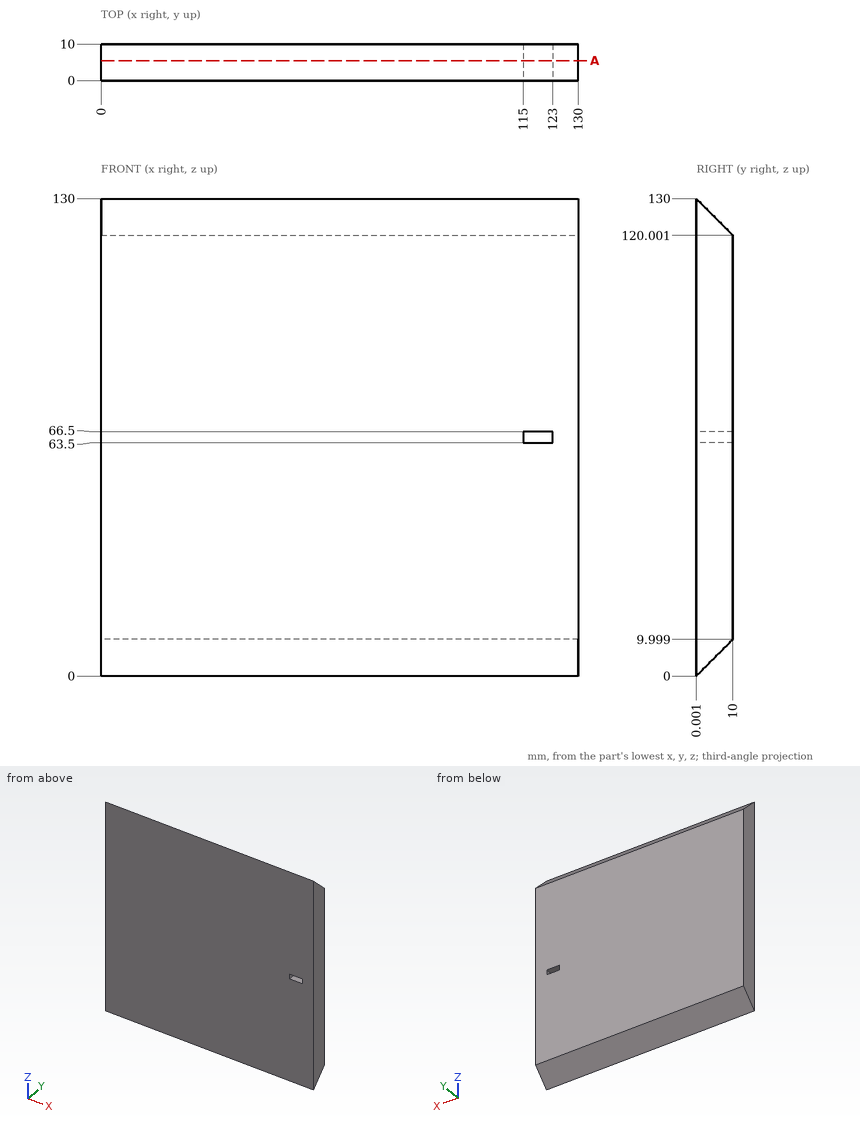
Verification items for this drawing (mm, ordinates from the low corner). Give positions to 0.01 mm unless a question says otherwise; leave off trailing zeros. Write each loop counter-clockwise with the first axis right and the second up, starting at its lowest first coordinate (ties: lowest second). Pieces come first, ordered by that corner, then holes.
1) Material ranges on L1, parallel to X at y = 7.25, z = 65; L2, parallel to Z at x = 91, y = 4.75; L3, parallel to Z at x = 116.5, y = 4, recorded low to high.
2) Gauge pin test, flat ends, axial feed: pin 1 (6 mm diameter, centred on y = 8, z = 87, fed in from -X); pin 2 (2.5 mm diameter, centred on x = 118.5, y = 3, fed in from +Z). Record the tip position at first contact, or that the pin passes through.
3) Section check A-A, the plane y = 5.5. Record the boundary of the cut face in (x, z).
Computed:
1. L1: x = 0 to 115, 123 to 130
1. L2: z = 4.75 to 125.25
1. L3: z = 4 to 63.5, 66.5 to 126
2. pin 1: stops at x = 0
2. pin 2: stops at z = 128.25
3. outline: (0, 5.5) - (130, 5.5) - (130, 124.5) - (0, 124.5) - close; hole (115, 63.5) - (123, 63.5) - (123, 66.5) - (115, 66.5) - close
